The model under review builds one solid part; all positions refer to its coordinate system, in mm. Give positions to 0.01 mm unless a question says otherwise; leave off trailing zeros. Write item = value, one per line. Start each with the question number.
1. Wall thickness on line 1 along X through (y, z) = (18, -24); line 2 along Y through (x, z) = (-6, -24.25); line 3 along X through (y, z) = (65.5, -24.75): over which ranges is each line inside the solid? List them lowest first. Write a range as from..to.
2. For pin 1 (2.5 mm diameter, centred on x = -11.58, y = -12.84, fed in from -Z); pin 2 (1.7 mm diameter, centred on x = -115.5, y = 65, fed in from -Z), all flat-tipped, find the tip position at first contact; note any pin that passes through.
3. We need section A-A on z = -24.5. Count the separate pieces of the cut face and the enclosed holes in it, then the cut area to 3 significant figures.
from build123d import *

# Parameters (mm, degrees)
SKETCH008_W     = 152.4
SKETCH008_H     = 127
SKETCH008_R     = 2.2606
PAD006_DEPTH    = 6.35
SKETCH097_R     = 1.778
POCKET025_DEPTH = 15.876
SKETCH098_R     = 1.5
POCKET037_DEPTH = 6.351
SKETCH114_R     = 3.683
POCKET039_DEPTH = 4.318
SKETCH115_R     = 2.794
POCKET040_DEPTH = 3.048


with BuildPart() as part:
    # Sketch008 → Pad006 (new body)
    with BuildSketch(Plane.XY):
        Rectangle(SKETCH008_W, SKETCH008_H)
        with Locations((-38.1, 58.7375)):
            Circle(SKETCH008_R, mode=Mode.SUBTRACT)
        with Locations((38.1, 58.7375)):
            Circle(SKETCH008_R, mode=Mode.SUBTRACT)
        with Locations((71.4375, 38.1)):
            Circle(SKETCH008_R, mode=Mode.SUBTRACT)
        with Locations((71.4375, -38.1)):
            Circle(SKETCH008_R, mode=Mode.SUBTRACT)
        with Locations((38.1, -58.7375)):
            Circle(SKETCH008_R, mode=Mode.SUBTRACT)
        with Locations((-38.1, -58.7375)):
            Circle(SKETCH008_R, mode=Mode.SUBTRACT)
        with Locations((-71.4375, -38.1)):
            Circle(SKETCH008_R, mode=Mode.SUBTRACT)
        with Locations((-71.4375, 38.1)):
            Circle(SKETCH008_R, mode=Mode.SUBTRACT)
    extrude(amount=PAD006_DEPTH)

    # Sketch097 (on Face2 of Pad032) → Pocket025 (cut, through all)
    with BuildSketch(Plane.YX.offset(9.525)):
        with Locations((31.75, 60.325)):
            Circle(SKETCH097_R)
        with Locations((31.75, 47.625)):
            Circle(SKETCH097_R)
        with Locations((0, 60.325)):
            Circle(SKETCH097_R)
        with Locations((0, 47.625)):
            Circle(SKETCH097_R)
        with Locations((0, -47.625)):
            Circle(SKETCH097_R)
        with Locations((31.75, -47.625)):
            Circle(SKETCH097_R)
        with Locations((0, -60.325)):
            Circle(SKETCH097_R)
        with Locations((31.75, -60.325)):
            Circle(SKETCH097_R)
    extrude(amount=-POCKET025_DEPTH, mode=Mode.SUBTRACT)

    # Sketch098 (on Face5 of Pocket025) → Pocket037 (cut, through all)
    with BuildSketch(Plane.XY.offset(6.35)):
        with Locations((23.193423, -15.40673)):
            Circle(SKETCH098_R)
        with Locations((55.193423, -15.40673)):
            Circle(SKETCH098_R)
        with Locations((55.193423, -47.40673)):
            Circle(SKETCH098_R)
        with Locations((23.193423, -47.40673)):
            Circle(SKETCH098_R)
    extrude(amount=-POCKET037_DEPTH, mode=Mode.SUBTRACT)

    # Sketch114 → Pocket039 (cut)
    with BuildSketch(Plane.XY):
        with Locations((-38.1, 58.7375)):
            Circle(SKETCH114_R)
        with Locations((38.1, 58.7375)):
            Circle(SKETCH114_R)
        with Locations((71.4375, 38.1)):
            Circle(SKETCH114_R)
        with Locations((71.4375, -38.1)):
            Circle(SKETCH114_R)
        with Locations((38.1, -58.7375)):
            Circle(SKETCH114_R)
        with Locations((-38.1, -58.7375)):
            Circle(SKETCH114_R)
        with Locations((-71.4375, -38.1)):
            Circle(SKETCH114_R)
        with Locations((-71.4375, 38.1)):
            Circle(SKETCH114_R)
    extrude(amount=POCKET039_DEPTH, mode=Mode.SUBTRACT)

    # Sketch115 (on Face4 of Pocket039) → Pocket040 (cut)
    with BuildSketch(Plane.YX):
        with Locations((31.75, 60.325)):
            Circle(SKETCH115_R)
        with Locations((31.75, 47.625)):
            Circle(SKETCH115_R)
        with Locations((0, 60.325)):
            Circle(SKETCH115_R)
        with Locations((0, 47.625)):
            Circle(SKETCH115_R)
        with Locations((0, -47.625)):
            Circle(SKETCH115_R)
        with Locations((31.75, -47.625)):
            Circle(SKETCH115_R)
        with Locations((0, -60.325)):
            Circle(SKETCH115_R)
        with Locations((31.75, -60.325)):
            Circle(SKETCH115_R)
    extrude(amount=-POCKET040_DEPTH, mode=Mode.SUBTRACT)


with BuildPart() as part_1:
    # Body006 placement: moved
    add(part.part.moved(Location((-66.7766, 34.5694, -25.6794))))


solid = part_1.part
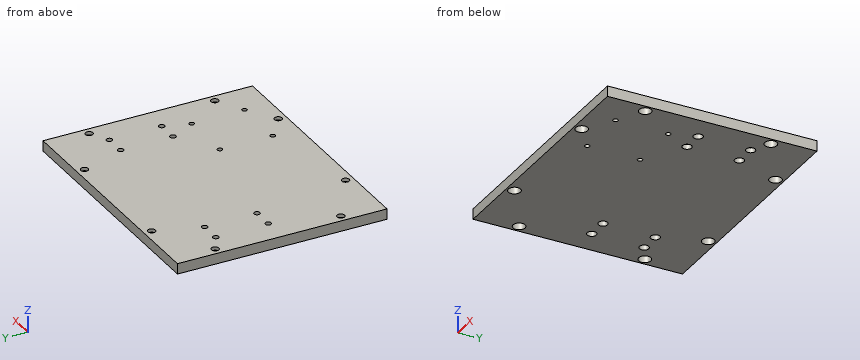
Final values:
q1.line_1 = -142.98..-44.53, -42.64..-12.53, -10.64..9.42
q1.line_2 = -28.93..31.81, 37.33..63.56, 69.08..98.07
q1.line_3 = -142.98..-129.77, -124.43..-117.07, -111.73..-21.82, -16.48..-9.12, -3.78..9.42
q2.pin_1 = through
q2.pin_2 = -22.63
q3.separate_pieces = 1
q3.enclosed_holes = 20
q3.area = 18,800 mm²
